Answer from the drawing. Dimensions are ordinates in mm from the lowest x, y and z of the part. Round coordinates to 2 decimals unless told otherwise and drop trailing zeros. Write each loop counter-clockwise with the first axis right and the second up, starting at its lowest first coordinate (ties: lowest second). Pieces come first, ordered by that corner, then holes. Notation, with made-up numbers: (7, 11.25) - (47, 11.25) arc R11 cw to (47, 29.25) - close; hole circle Ø1 at (38.25, -37). An arc over 180 degrees is marked (long way). One line per item, written item: value. Start each with the question number.
(1) A cutting plane is placed at A-A, the plane x = 196.2. Determine the outline of the cut face in (y, z), plus the area to 3 significant figures.
(2) A cutting plane is placed at B-B, the plane z = 25. Determine the outline of the cut face in (x, y), plus the area to 3 significant figures.
(3) Find the intervals of material crossed by L1, parallel to Z at x = 21, y = 3.3; L2, parallel to X at y = 1.4, z = 76.6; L3, parallel to X at y = 2.2, z = 75, in increasing order.
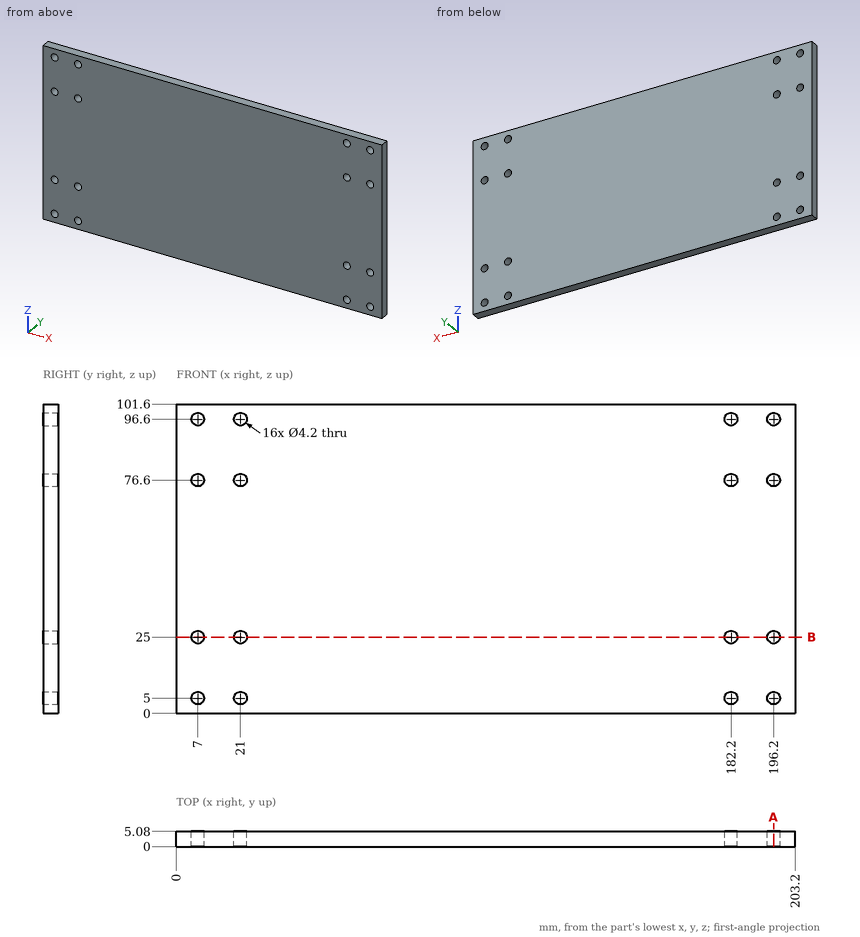
Here are the results:
1. outline: (0, 0) - (5.08, 0) - (5.08, 2.9) - (0, 2.9) - close; (0, 7.1) - (5.08, 7.1) - (5.08, 22.9) - (0, 22.9) - close; (0, 27.1) - (5.08, 27.1) - (5.08, 74.5) - (0, 74.5) - close; (0, 78.7) - (5.08, 78.7) - (5.08, 94.5) - (0, 94.5) - close; (0, 98.7) - (5.08, 98.7) - (5.08, 101.6) - (0, 101.6) - close
1. area: 431 mm²
2. outline: (0, 0) - (4.9, 0) - (4.9, 5.08) - (0, 5.08) - close; (9.1, 0) - (18.9, 0) - (18.9, 5.08) - (9.1, 5.08) - close; (23.1, 0) - (180.1, 0) - (180.1, 5.08) - (23.1, 5.08) - close; (184.3, 0) - (194.1, 0) - (194.1, 5.08) - (184.3, 5.08) - close; (198.3, 0) - (203.2, 0) - (203.2, 5.08) - (198.3, 5.08) - close
2. area: 947 mm²
3. L1: 0 to 2.9, 7.1 to 22.9, 27.1 to 74.5, 78.7 to 94.5, 98.7 to 101.6
3. L2: 0 to 4.9, 9.1 to 18.9, 23.1 to 180.1, 184.3 to 194.1, 198.3 to 203.2
3. L3: 0 to 5.64, 8.36 to 19.64, 22.36 to 180.84, 183.56 to 194.84, 197.56 to 203.2
